The listing builds one solid part. Answer for the finished solid, in the listing's coordinates (mm). A direction names the side the tool comes from. Give positions to 0.01 mm unless a question says otherwise; leave off trailing zeros. Loops run counter-clockwise (first coordinate to the right, second up) from the corner with the lowest first, then second, coordinate; pieces in that order, holes last. Notation, with made-up numbers: M 53.25,28.5 L 91.25,28.5 A18 cw 91.25,34.5 Z; hole C 78,-35 d3. An arc over 180 degrees is marked long. One line per item, written item: value. Start each with the question number.
Q1. Consider L1, parallel to X at y = 413, z = 9; L2, parallel to Y at x = 712, z = 5.6; L3, parallel to X at y = 379.5, z = 9.2. Determine where each line is inside the solid, lowest interval first.
Q2. The mould has two halves that part along Y. Classify faces 1 (the cylindrical face through (709.054, 339.277, 7.958)), 2 (the cylindrical face through (720.99, 330.85, 7.96)), 3 (the flat face through (704.7, 376.2, 11)): +Y half, -Y half, draft (parallel to the pull), parting line (faces both ways), or undercut.
Q3. For faces 4 (the flat face through (715, 378.5, 8)), 5 (the cylindrical face through (703.905, 371.475, 8.042)), determine the directions among +Z, -Z, +X, -X, +Y, -Y from which every point of the face is accessible in a straight line to the end or side of a thin tool.
Q4. Flat-ended cylindrical pins translate along their axes: pin 1 (2.5 mm diameter, centred on y = 375, z = 7.5, fed in from +X); pin 2 (1.8 mm diameter, centred on x = 716.5, z = 8, fed in from -Y); pin 3 (11 mm diameter, centred on x = 705, y = 338, fed in from -Z). Find the tip coordinate at first contact, or state that the pin passes through.
Q5. A cutting plane is placed at B-B, the plane z = 8.15. Determine the outline of the cut face in (x, y).
Q6. A cutting plane is placed at C-C, the plane x = 721. Determine the outline of the cut face in (y, z), and give its area (3 significant figures).
Q7. A cutting plane is placed at A-A, the plane x = 712. Determine the outline of the cut face in (y, z), and give its area (3 significant figures).
from build123d import *

# Parameters (mm, degrees)
BOSS_EXTRUDE1_START = 5
SKETCH1_R           = 4.25
BOSS_EXTRUDE1_DEPTH = 6
SKETCH3_R           = 1.5
CUT_EXTRUDE1_DEPTH  = 839.535032065


with BuildPart() as part:
    # Sketch1 → Boss-Extrude1 (new body)
    with BuildSketch(Plane.XY.offset(BOSS_EXTRUDE1_START)):
        with BuildLine():
            Line((724, 378.5), (724, 413))
            ThreePointArc((724, 413), (721.071067812, 420.071067812), (714, 423))
            Line((714, 423), (696, 423))
            ThreePointArc((696, 423), (688.928932188, 420.071067812), (686, 413))
            Line((686, 413), (686, 338))
            ThreePointArc((686, 338), (688.928932188, 330.928932188), (696, 328))
            Line((696, 328), (714, 328))
            ThreePointArc((714, 328), (721.071067812, 330.928932188), (724, 338))
            Line((724, 338), (724, 372.5))
            Line((724, 372.5), (705, 372.5))
            Line((705, 372.5), (705, 378.5))
            Line((705, 378.5), (724, 378.5))
        make_face()
        with Locations((705, 338)):
            Circle(SKETCH1_R, mode=Mode.SUBTRACT)
        with Locations((705, 413)):
            Circle(SKETCH1_R, mode=Mode.SUBTRACT)
    extrude(amount=BOSS_EXTRUDE1_DEPTH)

    # Sketch3 → Cut-Extrude1 (cut, through all)
    with BuildSketch(Plane.XY.offset(11)):
        with Locations((705, 378.5)):
            Circle(SKETCH3_R)
        with Locations((705, 372.5)):
            Circle(SKETCH3_R)
    extrude(amount=-CUT_EXTRUDE1_DEPTH, mode=Mode.SUBTRACT)


solid = part.part
Answer block:
1. L1: 686 to 700.75, 709.25 to 724
1. L2: 328 to 372.5, 378.5 to 423
1. L3: 686 to 703.88, 706.12 to 724
2. face 1: undercut
2. face 2: -Y half
2. face 3: draft
3. face 4: +Z, -Z, +X
3. face 5: +Z, -Z
4. pin 1: x = 705
4. pin 2: y = 328.13
4. pin 3: z = 5
5. outline: M 686,338 A10 ccw 696,328 L 714,328 A10 ccw 724,338 L 724,372.5 L 706.5,372.5 A1.5 cw long 705,374 L 705,377 A1.5 cw long 706.5,378.5 L 724,378.5 L 724,413 A10 ccw 714,423 L 696,423 A10 ccw 686,413 Z; hole C 705,338 d8.5; hole C 705,413 d8.5
6. outline: M 330.86,5 L 372.5,5 L 372.5,11 L 330.86,11 Z; M 378.5,5 L 420.14,5 L 420.14,11 L 378.5,11 Z
6. area: 500 mm^2
7. outline: M 328,5 L 372.5,5 L 372.5,11 L 328,11 Z; M 378.5,5 L 423,5 L 423,11 L 378.5,11 Z
7. area: 534 mm^2
